Build history of the part. All positions in model axes, mm. A direction names the side the tool comes from. Coordinates: 2 decimals unless noted, no trailing zeros. Order: outer loops, then holes, each group sorted by start corner. A loop starts at its lowest first (then second) coordinate and runs counter-clockwise, first axis right, second up. Notation, with made-up numbers: M 24,-26 L 48,-26 A16 cw 48,-1 Z; hole C 36.5,-24.5 d8. An arc over 180 degrees is marked long. Write item = value, one per line. Start each with the question number.
Q1. Band-saw the part on C-C on x = 18.5. Write the cut outline in (y, z), plus the area to 3 significant figures.
Q2. Pull direction X, two halves, no side cores. Call faces 1 (the face through (56.07, 0.99, -39.48)), 2 (the face through (12, 5.1, -13.4)), 3 (the face through (40, 12, -15)), 4 (the face through (2, 6, -35)): released by +X, released by -X, zero draft, split by the parting line, or undercut.
Q3. 3-axis set-ups, long thin cutter, end or side, ignore diameter. For faces 5 (the face through (5, 7, -6.8)), 6 (the face through (30.5, 6, -20)), 7 (the face through (-1, 2, -11)), 8 (the face through (16, 6, -34.46)): which of +Z, -Z, +X, -X, +Y, -Y reach the whole face in a straight line?
Q4. Band-saw the part on A-A on z = -11.3. Write the cut outline in (x, y).
Q5. Band-saw the part on B-B on y = 19.25. Write the cut outline in (x, z).
Q6. Band-saw the part on D-D on y = 3.75. Write the cut outline in (x, z).
Q7. Drill centre lines: probe 1 along Z at (x, y) = (24.5, 8.25); probe 2 along Y at (x, z) = (4, -11); probe 3 along X at (y, z) = (1.2, -50.8). Where is each one in solid material? Low to high.
Q8. Pin check, flat tips, straight feed: P1, Ø3, axis at y = 9.5, z = -45, coming from the +X side; P2, Ø6, axis at x = 29.5, y = 10, coming from the -Z side; P3, Ø6.5, axis at x = 54.4, z = -8, coming from the +Y side. Stop position of each tip, or through.
```python
from build123d import *

# Parameters (mm, degrees)
SKETCH1_R           = 2
BOSS_EXTRUDE1_DEPTH = 2
SKETCH2_W           = 28.5
SKETCH2_H           = 2
BOSS_EXTRUDE2_DEPTH = 9
LPATTERN1_COUNT     = 2
LPATTERN1_PITCH     = 15
SKETCH3_W           = 20
SKETCH3_H           = 8
BOSS_EXTRUDE3_DEPTH = 20
SKETCH4_W           = 48
SKETCH4_H           = 8
BOSS_EXTRUDE4_DEPTH = 20
SKETCH5_W           = 9
SKETCH5_H           = 11
SKETCH5_R           = 3.5
BOSS_EXTRUDE5_DEPTH = 14


with BuildPart() as part:
    # Sketch1 → Boss-Extrude1 (new body)
    with BuildSketch(Plane(origin=(0, 0, 0), x_dir=(1, 0, 0), z_dir=(0, 1, 0))):
        Polygon((54.8, 40.7), (54.8, 53.3), (0, 53.3), (0, 0), (54.8, 0), (54.8, 2.695833333), (57.3, 5.3), (57.3, 38.3), align=None)
        with Locations(Location((3, 3, 0), (0, 0, 270))):
            Circle(SKETCH1_R, mode=Mode.SUBTRACT)
        with Locations(Location((54.4, 8, 0), (0, 0, 270))):
            Circle(SKETCH1_R, mode=Mode.SUBTRACT)
        with Locations(Location((4, 50.8, 0), (0, 0, 270))):
            Circle(SKETCH1_R, mode=Mode.SUBTRACT)
        with Locations(Location((54.4, 35.5, 0), (0, 0, 270))):
            Circle(SKETCH1_R, mode=Mode.SUBTRACT)
    extrude(amount=BOSS_EXTRUDE1_DEPTH)

    # Sketch2 → Boss-Extrude2 (add)
    with BuildSketch(Plane(origin=(0, 2, 0), x_dir=(1, 0, 0), z_dir=(0, 1, 0))):
        with Locations((16.25, 35.460185898)):
            Rectangle(SKETCH2_W, SKETCH2_H)
    boss_extrude2 = extrude(amount=BOSS_EXTRUDE2_DEPTH)

    # LPattern1: Boss-Extrude2 ×2
    with Locations(*[(0, 0, i * LPATTERN1_PITCH) for i in range(1, LPATTERN1_COUNT)]):
        add(boss_extrude2)

    # Sketch3 → Boss-Extrude3 (add)
    with BuildSketch(Plane(origin=(0, 2, 0), x_dir=(1, 0, 0), z_dir=(0, 1, 0))):
        with Locations((40.3, 11)):
            Rectangle(SKETCH3_W, SKETCH3_H)
    extrude(amount=BOSS_EXTRUDE3_DEPTH)

    # Sketch4 → Boss-Extrude4 (add)
    with BuildSketch(Plane(origin=(0, 2, 0), x_dir=(1, 0, 0), z_dir=(0, 1, 0))):
        with Locations((26.8, 44.3)):
            Rectangle(SKETCH4_W, SKETCH4_H)
    extrude(amount=BOSS_EXTRUDE4_DEPTH)

    # Sketch5 → Boss-Extrude5 (add)
    with BuildSketch(Plane.ZY.offset(2)):
        with Locations((-11.3, 7.5)):
            Rectangle(SKETCH5_W, SKETCH5_H)
        with Locations((-11.3, 8.2)):
            Circle(SKETCH5_R, mode=Mode.SUBTRACT)
    extrude(amount=-BOSS_EXTRUDE5_DEPTH)


solid = part.part
```
Recorded:
q1.outline = M 0,-53.3 L 2,-53.3 L 2,-48.3 L 22,-48.3 L 22,-40.3 L 2,-40.3 L 2,-36.46 L 11,-36.46 L 11,-34.46 L 2,-34.46 L 2,-21.46 L 11,-21.46 L 11,-19.46 L 2,-19.46 L 2,0 L 0,0 Z
q1.area = 303 mm2
q2.face_1 = released by +X
q2.face_2 = undercut
q2.face_3 = zero draft
q2.face_4 = released by -X
q3.face_5 = +Z, +X, -X, +Y
q3.face_6 = +X, +Y
q3.face_7 = +Z, -Z, -X, -Y
q3.face_8 = +X, -X, +Y
q4.outline = M -2,2 L 0,2 L 0,0 L 57.3,0 L 57.3,2 L 50.3,2 L 50.3,22 L 30.3,22 L 30.3,2 L 12,2 L 12,4.7 L -2,4.7 Z; M -2,11.7 L 12,11.7 L 12,13 L -2,13 Z
q5.outline = M 2.8,-48.3 L 50.8,-48.3 L 50.8,-40.3 L 2.8,-40.3 Z; M 30.3,-15 L 50.3,-15 L 50.3,-7 L 30.3,-7 Z
q6.outline = M -2,-15.8 L 12,-15.8 L 12,-6.8 L -2,-6.8 Z; M 2,-36.46 L 30.5,-36.46 L 30.5,-34.46 L 2,-34.46 Z; M 2,-21.46 L 30.5,-21.46 L 30.5,-19.46 L 2,-19.46 Z; M 2.8,-48.3 L 50.8,-48.3 L 50.8,-40.3 L 2.8,-40.3 Z; M 30.3,-15 L 50.3,-15 L 50.3,-7 L 30.3,-7 Z
q7.probe_1 = -48.3 to -40.3, -36.46 to -34.46, -21.46 to -19.46
q7.probe_2 = 0 to 4.71, 11.69 to 13
q7.probe_3 = 0 to 2, 6 to 54.8
q8.P1 = 50.8
q8.P2 = -48.3
q8.P3 = 2
